CAD build for the part. Positions are in the model's coordinates, mm. Face numbers are marked on the shaded views. A direction names the side the tool comes from. Give positions to 0.01 mm unless a question says otherwise; leave off trailing zeros. Write each loop counter-clockwise with the first axis right and the second up, starting at its lowest first coordinate (ties: lowest second). Pieces come first, ordered by that corner, then holes. Notation, with made-up numbers: (-11, 23) - (5, 23) arc R14 ccw to (5, 45) - close; hole circle Ø7 at (-15, -10). An arc over 180 degrees is marked (long way). Answer as a JSON object with one key per item and string values.
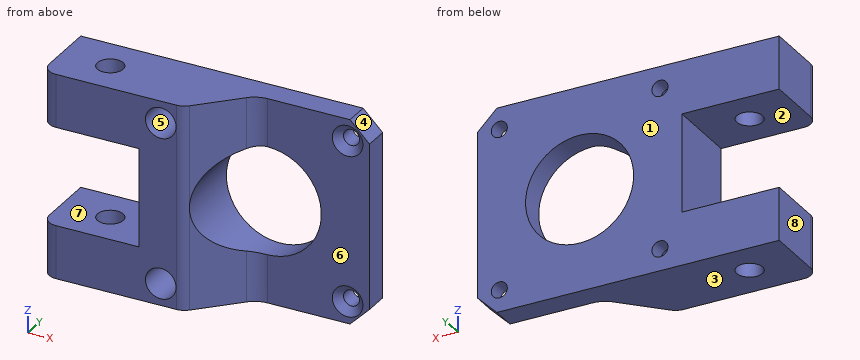
Autodesk Inventor part; units mm, degrees
ref_plane "YZ Plane" through (0, 0, 0) normal (1, 0, 0) x (0, 1, 0)
ref_plane "XZ Plane" through (0, 0, 0) normal (0, 1, 0) x (-1, 0, 0)
ref_plane "XY Plane" through (0, 0, 0) normal (0, 0, 1) x (1, 0, 0)
sketch "Boceto1" plane through (0, 0, 0) normal (0, 1, 0) x (-1, 0, 0)
  line L0 (-21, 21) -> (21, 21)
  line L1 (21, 21) -> (21, -21)
  line L2 (21, -21) -> (-21, -21)
  line L3 (-21, -21) -> (-21, 21)
  line L4 (-21, 21) -> (21, -21) construction
  line L5 (21, 21) -> (-21, -21) construction
  circle A0 centre (0, 0) radius 11.1
  dimension "d0" = 42
  dimension "d1" = 42
  dimension "d2" = 22.2
extrude "Extrusión1" add sketch "Boceto1" along normal blind 5
sketch "Boceto3" plane through (0, 0, 0) normal (0, -1, 0) x (1, 0, 0)
  circle A0 centre (16.5, 16.5) radius 1.65
  point P0 (0, 0)
  dimension "d9" = 3.3
  dimension "d10" = 16.5
  dimension "d11" = 16.5
extrude "Extrusión3" cut sketch "Boceto3" against normal through all
chamfer "Chaflán1" distance 1.5 angle 45 1 edges at (14.85, 0, 16.5)
pattern_circular "Patrón circular1" count 4 over 360 about axis through (0, 0, 0) along (0, 1, 0) of "Extrusión3", "Chaflán1"
chamfer "Chaflán3" distance 4 angle 45 2 edges at (21, 2.5, -21) (21, 2.5, 21)
sketch "Boceto4" plane through (0, 0, 0) normal (0, -1, 0) x (1, 0, 0)
  circle A0 centre (-16.5, 16.5) radius 3.15
  circle A1 centre (-16.5, 16.5) radius 1.65
  circle A2 centre (-16.5, -16.5) radius 1.65
  circle A3 centre (-16.5, -16.5) radius 3.15
  line L0 (-21, -21) -> (-21, 21)
  line L1 (17, -21) -> (-21, -21)
  line L2 (-21, 21) -> (-12, 21)
  line L3 (-12, 21) -> (-12, -21)
  line L4 (-12, -21) -> (-21, -21)
  line L5 (-21, -21) -> (-21, 21)
  point P0 (0, 0)
  dimension "d27" = 9
extrude "Extrusión4" add sketch "Boceto4" along normal blind 10 contours L0 L2 L3 L1
sketch "Boceto5" plane through (0, -10, 0) normal (0, -1, 0) x (1, 0, 0)
  line L0 (-21, -21) -> (-21, 21)
  line L1 (-21, 21) -> (-41, 21)
  line L2 (-41, 21) -> (-41, -21)
  line L3 (-41, -21) -> (-21, -21)
  line L4 (-21, -21) -> (-21, 21)
  line L5 (-21, 10.1) -> (-41, 10.1)
  line L6 (-41, 10.1) -> (-41, -10.1)
  line L7 (-41, -10.1) -> (-21, -10.1)
  line L8 (-21, -10.1) -> (-21, 10.1)
  line L9 (-31, 10.1) -> (-31, 21)
  line L10 (-31, -10.1) -> (-31, -21)
  line L11 (-21, -21) -> (-12, -21)
  point P0 (0, 0)
  dimension "d30" = 20.2
  dimension "d31" = 20
extrude "Extrusión5" add sketch "Boceto5" against normal up to surface (15 mm away) contours L3 L10 L7 L0 | L3 L2 L7 L10 | L5 L9 L1 L0 | L5 L2 L1 L9
chamfer "Chaflán4" distance 10 angle 45 1 edges at (-12, 0, 0)
fillet "Empalme2" radius 5 2 edges at (-2, 0, -15.9592) (-2, 0, 15.9592)
fillet "Empalme3" radius 3 1 edges at (-12, -10, 0)
fillet "Empalme4" radius 3 2 edges at (-41, -10, 15.55) (-41, -10, -15.55)
sketch "Boceto6" plane through (17, 0, -21) normal (0, 0, -1) x (-1, 0, 0)
  circle A0 centre (47.9, -2.5) radius 2.65
  line L0 (0, 5) -> (58, 5)
  line L1 (58, -7) -> (58, 5)
  point P0 (17, 0)
  dimension "d40" = 7.5
  dimension "d41" = 10.1
  dimension "d42" = 5.3
extrude "Extrusión6" cut sketch "Boceto6" against normal through all
properties part number "Zmotorsupport"
(1) 3-axis set-ups, long thin cutter, end or side, ignore diameter. For the marked faces 4, 5, 6, 7 and 8: which of +Z, -Z, +X, -X, +Y, -Y reach the whole face in a straight line?
Answer key:
{"face 4": "+Z, +X, +Y, -Y", "face 5": "-Y", "face 6": "+Z, -Z, +X, -Y", "face 7": "-X, +Y, -Y", "face 8": "+Z, -Z, -X, +Y, -Y"}
(2) Saw through at C-C, the plane x = -30.9. Give the cut face in (y, z).
Answer key:
{"outline": "(-10, -21) - (-5.15, -21) - (-5.15, -10.1) - (-10, -10.1) - close; (-10, 10.1) - (-5.15, 10.1) - (-5.15, 21) - (-10, 21) - close; (0.15, -21) - (5, -21) - (5, -10.1) - (0.15, -10.1) - close; (0.15, 10.1) - (5, 10.1) - (5, 21) - (0.15, 21) - close"}
(3) Flat gauge pins, fed straight in: P1, Ø5, axis at y = -5.5, z = 5.5, coming from the +X side; P2, Ø7.5, axis at y = -5.5, z = 0, coming from the -X side; P3, Ø3, axis at x = -30.9, y = -2.5, coming from the -Z side; P4, Ø5, axis at y = -7.5, z = -7.5, coming from the +X side. Where does each tip first touch, or does it go through?
Answer key:
{"P1": "stops at x = -7.69", "P2": "stops at x = -21", "P3": "passes through", "P4": "stops at x = -7.19"}
(4) Pull direction Z, two halves, no side cores. Call the marked faces 1, 2 and 3: pulls with the +Z half, pulls with the -Z half, needs draft (parallel to the pull), parting line crosses it, or undercut.
Answer key:
{"face 1": "needs draft", "face 2": "undercut", "face 3": "pulls with the -Z half"}
(5) Saw through at D-D, the plane z = 3. Give the cut face in (x, y), and give its area (3 significant figures).
Answer key:
{"outline": "(-21, -10) - (-13.24, -10) arc R3 ccw to (-11.12, -9.12) - (-10.69, -8.69) - (-10.69, 5) - (-21, 5) - close; (10.69, 0) - (21, 0) - (21, 5) - (10.69, 5) - close", "area": "205 mm²"}
(6) Saw through at B-B, the plane y = -3.75. Give the cut face in (x, z), and give its area (3 significant figures).
Answer key:
{"outline": "(-41, -21) - (-33.24, -21) - (-33.24, -10.1) - (-41, -10.1) - close; (-41, 10.1) - (-33.24, 10.1) - (-33.24, 21) - (-41, 21) - close; (-28.56, -21) - (-5.75, -21) - (-5.75, -9.49) arc R11.1 cw to (-5.75, 9.49) - (-5.75, 21) - (-28.56, 21) - (-28.56, 10.1) - (-21, 10.1) - (-21, -10.1) - (-28.56, -10.1) - close; hole circle Ø6.3 at (-16.5, -16.5); hole circle Ø6.3 at (-16.5, 16.5)", "area": "840 mm²"}
(7) Saw through at A-A, the plane x = -16.5. Give the cut face in (y, z).
Answer key:
{"outline": "(-10, -21) - (5, -21) - (5, -18.15) - (1.5, -18.15) - (0, -19.65) - (-10, -19.65) - close; (-10, -13.35) - (0, -13.35) - (1.5, -14.85) - (5, -14.85) - (5, 14.85) - (1.5, 14.85) - (0, 13.35) - (-10, 13.35) - close; (-10, 19.65) - (0, 19.65) - (1.5, 18.15) - (5, 18.15) - (5, 21) - (-10, 21) - close"}
(8) Probe L1, parallel to Z at x = -21.5, y = -3.5; L2, parallel to Z at x = -16.5, y = 3.9; L3, parallel to X at y = 0.25, z = 0. List the from-to ranges inside material, lowest first. Write a range as [from, to].
Answer key:
{"L1": "z = [-21, -10.1], [10.1, 21]", "L2": "z = [-21, -18.15], [-14.85, 14.85], [18.15, 21]", "L3": "x = [-21, -11.1], [11.1, 21]"}
